Build history of the part. All positions in model axes, mm. Round coordinates to 2 decimals unless told otherwise and drop trailing zeros. Loops run counter-clockwise (first coordinate to the right, second up) from the corner with the lowest first, then second, coordinate; pieces in that order, holes last. Notation, with made-up numbers: (57, 40.5) -> (107, 40.5) arc R26 cw to (107, 77.5) -> close; hole circle Ø3 at (29.5, 7.25). An arc over 180 degrees is marked (long way). Put each result on its own line as item: value. Start each with the question number.
Item 1: Cut at D-D, the plane x = 3. List the corners of the cut face in (y, z).
Item 2: Cut at B-B, the plane z = -11. List the corners of the cut face in (x, y), plus the area to 3 significant figures.
Item 3: Cut at A-A, the plane x = 36. List the corners of the cut face in (y, z).
Item 4: Cut at C-C, the plane y = -8. List the corners of the cut face in (x, z).
Item 5: Flat gauge pins, fed straight in: pin 1 Ø11 at (x, z) = (31.34, -9.86) entering from +Y; pin 2 Ø14.5 at (x, z) = (14.78, -7.5) entering from -Y. Where does each tip first touch, or does it go through?
Item 6: Drill centre lines: probe 1 along X at (y, z) = (-6.75, -7); probe 2 along X at (y, z) = (-2.75, -9); probe 3 along X at (y, z) = (-9.5, -15). Where is each one in solid material? Low to high. Write a range as [from, to].
Item 7: Pull direction Z, two halves, no side cores. Call faces 1 (the cylindrical face through (-19.84, -5.46, -3.6)), 2 (the flat face through (8, -2, -30.406)), 3 (the cylindrical face through (9.61, -9.14, 11.34)), 4 (the flat face through (8, 0, -8)): +Z half, -Z half, draft (parallel to the pull), parting line (faces both ways), or undercut.
```python
from build123d import *

# Parameters (mm, degrees)
F0_W     = 94.063151
F0_H     = 43.580622
F1_DEPTH = 11.07007
F2_R     = 6.969276
F2_R_2   = 4.505481
F2_R_3   = 8.13069
F2_R_4   = 7.123996
F3_DEPTH = 11.07007
F4_R     = 6.425985


with BuildPart() as f1:
    # F0 (on Front) → F1 (new body)
    with BuildSketch(Plane.XZ):
        with Locations((8.955018, -8.615909)):
            Rectangle(F0_W, F0_H)
    extrude(amount=F1_DEPTH)

    # F2 (on Front) → F3 (cut, through all)
    with BuildSketch(Plane.XZ):
        with Locations((31.341657, -9.856824)):
            Circle(F2_R)
        with Locations((14.776061, -7.497377)):
            Circle(F2_R_2)
        with Locations((-10.0703, -8.691281)):
            Circle(F2_R_3)
        with Locations((-26.636144, -5.740199)):
            Circle(F2_R_4)
    extrude(amount=F3_DEPTH, mode=Mode.SUBTRACT)

    # F4
    f4_edges = [f1.edges().sort_by_distance(p)[0] for p in [
        (8.955019, -11.07007, 13.174402),
        (8.955019, -11.07007, -30.40622),
    ]]
    fillet(f4_edges, radius=F4_R)


solid = f1.part
```
Reply:
1. outline: (-11.07, -23.98) arc R6.43 ccw to (-4.64, -30.41) -> (0, -30.41) -> (0, 13.17) -> (-4.64, 13.17) arc R6.43 ccw to (-11.07, 6.75) -> close
2. outline: (-38.08, -11.07) -> (-31.44, -11.07) -> (-31.44, 0) -> (-38.08, 0) -> close; (-21.83, -11.07) -> (-17.87, -11.07) -> (-17.87, 0) -> (-21.83, 0) -> close; (-2.27, -11.07) -> (11.94, -11.07) -> (11.94, 0) -> (-2.27, 0) -> close; (17.61, -11.07) -> (24.47, -11.07) -> (24.47, 0) -> (17.61, 0) -> close; (38.22, -11.07) -> (55.99, -11.07) -> (55.99, 0) -> (38.22, 0) -> close
2. area: 547 mm^2
3. outline: (-11.07, -23.98) arc R6.43 ccw to (-4.64, -30.41) -> (0, -30.41) -> (0, -15.04) -> (-11.07, -15.04) -> close; (-11.07, -4.67) -> (0, -4.67) -> (0, 13.17) -> (-4.64, 13.17) arc R6.43 ccw to (-11.07, 6.75) -> close
4. outline: (-38.08, -29.46) -> (55.99, -29.46) -> (55.99, 12.23) -> (-38.08, 12.23) -> close; hole circle Ø14.25 at (-26.64, -5.74); hole circle Ø16.26 at (-10.07, -8.69); hole circle Ø9.01 at (14.78, -7.5); hole circle Ø13.94 at (31.34, -9.86)
5. pin 1: passes through
5. pin 2: stops at y = -11.07
6. probe 1: x = [-38.08, -33.65], [-19.62, -18.02], [-2.12, 10.3], [19.25, 24.98], [37.7, 55.99]
6. probe 2: x = [-38.08, -32.97], [-20.3, -18.2], [-1.95, 10.53], [19.02, 24.43], [38.26, 55.99]
6. probe 3: x = [-38.08, -15.2], [-4.94, 26.64], [36.04, 55.99]
7. face 1: undercut
7. face 2: -Z half
7. face 3: +Z half
7. face 4: draft
